from build123d import *

# Parameters (mm, degrees)
ESQUISSE1_W             = 20
ESQUISSE1_H             = 20
BOSS_EXTRU_1_DEPTH      = 300
ESQUISSE2_R             = 3
ENL_V_MAT_EXTRU_1_DEPTH = 200
ENL_V_START             = -200
ESQUISSE3_R             = 3
ENL_V_MAT_EXTRU_2_DEPTH = 200


with BuildPart() as part:
    # Esquisse1 → Boss.-Extru.1 (new body)
    with BuildSketch(Plane.XY):
        Rectangle(ESQUISSE1_W, ESQUISSE1_H)
    extrude(amount=BOSS_EXTRU_1_DEPTH)

    # Esquisse2 → Enlèv. mat.-Extru.1 (cut)
    with BuildSketch(Plane.XY.offset(300)):
        Circle(ESQUISSE2_R)
    extrude(amount=-ENL_V_MAT_EXTRU_1_DEPTH, mode=Mode.SUBTRACT)

    # Esquisse3 → Enlèv. mat.-Extru.2 (cut)
    with BuildSketch(Plane(origin=(0, 0, 0), x_dir=(-1, 0, 0), z_dir=(0, 0, -1)).offset(ENL_V_START)):
        with Locations(Location((0, 0, 0), (0, 0, 180))):
            Circle(ESQUISSE3_R)
    extrude(amount=ENL_V_MAT_EXTRU_2_DEPTH, mode=Mode.SUBTRACT)


solid = part.part
Source: CAD feature listing. Evaluate the final solid. Frame: model axes, mm. Give positions to 0.01 mm unless a question says otherwise; leave off trailing zeros. Loops run counter-clockwise (first coordinate to the right, second up) from the corner with the lowest first, then second, coordinate; pieces in that order, holes last. Notation, with made-up numbers: (42, 25) -> (84, 25) arc R20 ccw to (84, 52) -> close; hole circle Ø2 at (-22, -34). An arc over 180 degrees is marked (long way). Use a Markdown table: item, result. Add a question column.
1) Line query: line 1 along Y through (x, z) = (0, 197); line 2 along X through (y, z) = (2.5, 238). Output: solid intervals per line, ascending. Write a range as [from, to].
2) Pull-direction query (X, two-part tool) for faces 1 (the face through (2.86, -0.9, 152.1)), 2 (the face through (0, -10, 148)), 3 (the face through (10, 0, 148)); classes: +X half, -X half, draft (parallel to the pull), parting line (faces both ways), or undercut.
3) Section query C-C, the plane z = 265. Return the cut outline in (x, y).
4) Section query A-A, the plane y = 0. Return the cut outline in (x, z).
Numbers:
| question | item | result |
|---|---|---|
| 1 | line 1 | y = [-10, -3], [3, 10] |
| 1 | line 2 | x = [-10, -1.66], [1.66, 10] |
| 2 | face 1 | undercut |
| 2 | face 2 | draft |
| 2 | face 3 | +X half |
| 3 | outline | (-10, -10) -> (10, -10) -> (10, 10) -> (-10, 10) -> close; hole circle Ø6 at (0, 0) |
| 4 | outline | (-10, 0) -> (-3, 0) -> (-3, 300) -> (-10, 300) -> close; (3, 0) -> (10, 0) -> (10, 300) -> (3, 300) -> close |
